```python
from build123d import *

# Parameters (mm, degrees)
ESTRUSIONE_ESTRUSIONE1_DEPTH = 11
SCHIZZO2_R                   = 6.35
ESTRUSIONE_ESTRUSIONE2_DEPTH = 1
SCHIZZO3_R                   = 5.499261314
ESTRUSIONE_ESTRUSIONE3_DEPTH = 1
FORO_0_6_0_6_1_D             = 6
FORO_0_6_0_6_1_DEPTH         = 13


with BuildPart() as part:
    # Schizzo1 → Estrusione-Estrusione1 (new body)
    with BuildSketch(Plane(origin=(0, 11, 0), x_dir=(1, 0, 0), z_dir=(0, 1, 0))):
        Polygon((-3.175, 5.499261314), (-6.35, 0), (-3.175, -5.499261314), (3.175, -5.499261314), (6.35, 0), (3.175, 5.499261314), align=None)
    extrude(amount=-ESTRUSIONE_ESTRUSIONE1_DEPTH)

    # Schizzo2 → Estrusione-Estrusione2 (add)
    with BuildSketch(Plane.XZ):
        Circle(SCHIZZO2_R)
    extrude(amount=ESTRUSIONE_ESTRUSIONE2_DEPTH)

    # Schizzo3 → Estrusione-Estrusione3 (add)
    with BuildSketch(Plane(origin=(0, 11, 0), x_dir=(-1, 0, 0), z_dir=(0, 1, 0))):
        Circle(SCHIZZO3_R)
    extrude(amount=ESTRUSIONE_ESTRUSIONE3_DEPTH)

    # Foro Ø0.6 (0.6)-1
    with Locations(Plane(origin=(0, -1, 0), x_dir=(-1, 0, 0), z_dir=(0, -1, 0))):
        with Locations((0, 0)):
            Hole(FORO_0_6_0_6_1_D / 2, depth=FORO_0_6_0_6_1_DEPTH)


solid = part.part
```
Verification items for the finished model (mm, model axes). A direction names the side the tool comes from. Coordinates: 2 decimals unless noted, no trailing zeros. Order: outer loops, then holes, each group sorted by start corner. A loop starts at its lowest first (then second) coordinate and runs counter-clockwise, first axis right, second up. Notation, with made-up numbers: (-16, -21) -> (6, -21) arc R9 ccw to (6, -5) -> close; hole circle Ø4 at (-16.75, 75.5). An arc over 180 degrees is marked (long way). Put each result on its own line as item: value. Start each with the question number.
1) Tool access check on faces 4 (the flat face through (-4.785, 5.577, 2.711)), 5 (the flat face through (3, 11, 5)), 6 (the flat face through (3, 11, -5)). Record the directions out of +Z, -Z, +X, -X, +Y, -Y that give a thin tool (end or side, any length) a straight path to the whole face; none if there is none.
2) Go/stop test with flat-tipped pins: pin 1 (7 mm diameter, centred on x = 1, y = 8, fed in from +Z); pin 2 (2 mm diameter, centred on y = 2, z = -5, fed in from +X); pin 3 (5 mm diameter, centred on x = 5, y = 8, fed in from -Z). Record where each tip stops, or that it passes through.
3) Cross-section at B-B (y = 10.75). Enter the section's corners in (x, z) (3 decimals), plus the area to 3 significant figures.
4) Cross-section at A-A (z = -1.75). Enter the section's corners in (x, y), plus the area to 3 significant figures.
5) Cross-section at D-D (z = -3.5). Enter the section's corners in (x, y).
6) Material ranges on L1, parallel to Z at x = 0, y = 6; L2, parallel to Z at x = 2, y = 7; L3, parallel to X at y = 5.75, z = 2.25, recorded low to high.
7) Cross-section at C-C (x = -3.75). Enter the section's corners in (y, z).
8) Release check for a two-part mould opening along Z. For faces 1 (the cylindrical face through (-3, 6, 0)), 2 (the flat face through (3, -1, -1)), 3 (the flat face through (-4.74, 5.58, -2.79)) record: pulls with the +Z half, pulls with the -Z half, needs draft (parallel to the pull), parting line crosses it, or undercut.
Geometry check:
1. face 4: +Z, -X, +Y
1. face 5: +Z, +X, +Y
1. face 6: -Z, +X, +Y
2. pin 1: stops at z = 5.5
2. pin 2: stops at x = 4.04
2. pin 3: stops at z = -5.5
3. outline: (-6.35, 0) -> (-3.175, -5.499) -> (3.175, -5.499) -> (6.35, 0) -> (3.175, 5.499) -> (-3.175, 5.499) -> close; hole circle Ø6 at (0, 0)
3. area: 76.5 mm^2
4. outline: (-6.1, -1) -> (-2.44, -1) -> (-2.44, 12) -> (-5.21, 12) -> (-5.21, 11) -> (-5.34, 11) -> (-5.34, 0) -> (-6.1, 0) -> close; (2.44, -1) -> (6.1, -1) -> (6.1, 0) -> (5.34, 0) -> (5.34, 11) -> (5.21, 11) -> (5.21, 12) -> (2.44, 12) -> close
4. area: 76.8 mm^2
5. outline: (-5.3, -1) -> (5.3, -1) -> (5.3, 0) -> (4.33, 0) -> (4.33, 11) -> (4.24, 11) -> (4.24, 12) -> (-4.24, 12) -> (-4.24, 11) -> (-4.33, 11) -> (-4.33, 0) -> (-5.3, 0) -> close
6. L1: z = -5.5 to -3, 3 to 5.5
6. L2: z = -5.5 to -2.24, 2.24 to 5.5
6. L3: x = -5.05 to -1.98, 1.98 to 5.05
7. outline: (-1, -5.12) -> (0, -5.12) -> (0, -4.5) -> (11, -4.5) -> (11, -4.02) -> (12, -4.02) -> (12, 4.02) -> (11, 4.02) -> (11, 4.5) -> (0, 4.5) -> (0, 5.12) -> (-1, 5.12) -> close
8. face 1: undercut
8. face 2: needs draft
8. face 3: pulls with the -Z half
